from build123d import *

# Parameters (mm, degrees)
F1_DEPTH = 4.7625
F2_R     = 10


# Not quite as in the source:
# - a feature names something its author has since deleted; it is built from what else it names


with BuildPart() as f1:
    # F0 (on Top) → F1 (new body)
    with BuildSketch(Plane.XY):
        with BuildLine():
            ThreePointArc((-6.35, 0), (-4.4901280605, 4.4901280605), (0, 6.35))
            Line((0, 6.35), (-12.4931629071, 6.35))
            ThreePointArc((-12.4931629071, 6.35), (-13.6287381062, 3.2648303256), (-14.0143362106, 0))
            Line((-14.0143362106, 0), (-6.35, 0))
        make_face()
        with BuildLine():
            ThreePointArc((0, 6.35), (4.4901280605, 4.4901280605), (6.35, 0))
            Line((6.35, 0), (14.0143362106, 0))
            ThreePointArc((14.0143362106, 0), (13.6287381062, 3.2648303256), (12.4931629071, 6.35))
            Line((12.4931629071, 6.35), (0, 6.35))
        make_face()
        with BuildLine():
            Line((12.4931629071, -6.35), (0, -6.35))
            Line((0, -6.35), (0, -14.0143362106))
            ThreePointArc((0, -14.0143362106), (7.3283894713, -11.9455567966), (12.4931629071, -6.35))
        make_face()
        with BuildLine():
            Line((0, -14.0143362106), (0, -6.35))
            Line((0, -6.35), (-12.4931629071, -6.35))
            ThreePointArc((-12.4931629071, -6.35), (-7.3283894713, -11.9455567966), (0, -14.0143362106))
        make_face()
        with BuildLine():
            Line((-12.4931629071, -6.35), (0, -6.35))
            ThreePointArc((0, -6.35), (-4.4901280605, -4.4901280605), (-6.35, 0))
            Line((-6.35, 0), (-14.0143362106, 0))
            ThreePointArc((-14.0143362106, 0), (-13.6287381062, -3.2648303256), (-12.4931629071, -6.35))
        make_face()
        with BuildLine():
            Line((-27.86051193, -6.35), (-12.4931629071, -6.35))
            ThreePointArc((-12.4931629071, -6.35), (-13.6287381062, -3.2648303256), (-14.0143362106, 0))
            Line((-14.0143362106, 0), (-28.575, 0))
            ThreePointArc((-28.575, 0), (-28.395816183, -3.1950349451), (-27.86051193, -6.35))
        make_face()
        with BuildLine():
            ThreePointArc((12.4931629071, 6.35), (13.6287381062, 3.2648303256), (14.0143362106, 0))
            Line((14.0143362106, 0), (28.575, 0))
            ThreePointArc((28.575, 0), (28.395816183, 3.1950349451), (27.86051193, 6.35))
            Line((27.86051193, 6.35), (12.4931629071, 6.35))
        make_face()
        with BuildLine():
            Line((0, 14.0143362106), (0, 6.35))
            Line((0, 6.35), (12.4931629071, 6.35))
            ThreePointArc((12.4931629071, 6.35), (7.3283894713, 11.9455567966), (0, 14.0143362106))
        make_face()
        with BuildLine():
            Line((-12.4931629071, 6.35), (0, 6.35))
            Line((0, 6.35), (0, 14.0143362106))
            ThreePointArc((0, 14.0143362106), (-7.3283894713, 11.9455567966), (-12.4931629071, 6.35))
        make_face()
        with BuildLine():
            Line((-24.9023895556, -14.0143362106), (0, -14.0143362106))
            ThreePointArc((0, -14.0143362106), (-7.3283894713, -11.9455567966), (-12.4931629071, -6.35))
            Line((-12.4931629071, -6.35), (-27.86051193, -6.35))
            ThreePointArc((-27.86051193, -6.35), (-26.6583280736, -10.2890315054), (-24.9023895556, -14.0143362106))
        make_face()
        with BuildLine():
            Line((24.9023895556, 14.0143362106), (0, 14.0143362106))
            ThreePointArc((0, 14.0143362106), (7.3283894713, 11.9455567966), (12.4931629071, 6.35))
            Line((12.4931629071, 6.35), (27.86051193, 6.35))
            ThreePointArc((27.86051193, 6.35), (26.6583280736, 10.2890315054), (24.9023895556, 14.0143362106))
        make_face()
        with BuildLine():
            Line((14.0143362106, 0), (6.35, 0))
            ThreePointArc((6.35, 0), (4.4901280605, -4.4901280605), (0, -6.35))
            Line((0, -6.35), (12.4931629071, -6.35))
            ThreePointArc((12.4931629071, -6.35), (13.6287381062, -3.2648303256), (14.0143362106, 0))
        make_face()
        with BuildLine():
            ThreePointArc((-14.0143362106, 0), (-13.6287381062, 3.2648303256), (-12.4931629071, 6.35))
            Line((-12.4931629071, 6.35), (-27.86051193, 6.35))
            ThreePointArc((-27.86051193, 6.35), (-28.395816183, 3.1950349451), (-28.575, 0))
            Line((-28.575, 0), (-14.0143362106, 0))
        make_face()
        with BuildLine():
            ThreePointArc((-12.4931629071, 6.35), (-7.3283894713, 11.9455567966), (0, 14.0143362106))
            Line((0, 14.0143362106), (-24.9023895556, 14.0143362106))
            ThreePointArc((-24.9023895556, 14.0143362106), (-26.6583280736, 10.2890315054), (-27.86051193, 6.35))
            Line((-27.86051193, 6.35), (-12.4931629071, 6.35))
        make_face()
        with BuildLine():
            Line((28.575, 0), (14.0143362106, 0))
            ThreePointArc((14.0143362106, 0), (13.6287381062, -3.2648303256), (12.4931629071, -6.35))
            Line((12.4931629071, -6.35), (27.86051193, -6.35))
            ThreePointArc((27.86051193, -6.35), (28.395816183, -3.1950349451), (28.575, 0))
        make_face()
        with BuildLine():
            ThreePointArc((12.4931629071, -6.35), (7.3283894713, -11.9455567966), (0, -14.0143362106))
            Line((0, -14.0143362106), (24.9023895556, -14.0143362106))
            ThreePointArc((24.9023895556, -14.0143362106), (26.6583280736, -10.2890315054), (27.86051193, -6.35))
            Line((27.86051193, -6.35), (12.4931629071, -6.35))
        make_face()
    extrude(amount=F1_DEPTH)

    # F2
    f2_edges = [f1.edges().sort_by_distance(p)[0] for p in [
        (24.90239, 14.014336, 2.38125),
        (-24.90239, 14.014336, 2.38125),
        (24.90239, -14.014336, 2.38125),
        (-24.90239, -14.014336, 2.38125),
    ]]
    fillet(f2_edges, radius=F2_R)


solid = f1.part
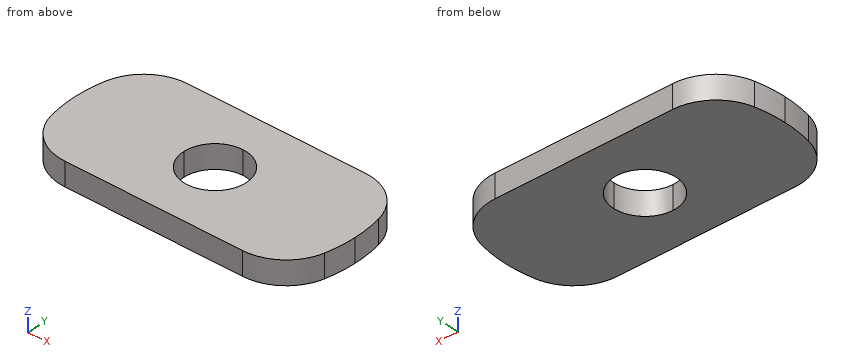
CAD build for the part. Positions are in the model's coordinates, mm. Coordinates: 2 decimals unless noted, no trailing zeros. Write each loop counter-clockwise with the first axis right and the second up, starting at its lowest first coordinate (ties: lowest second). Pieces come first, ordered by that corner, then holes. Notation, with made-up numbers: M 55.25,26 L 60.25,26 A26 ccw 60.25,65 Z; hole C 62.25,65.25 d5. An arc over 180 degrees is marked long. Return JSON: item names as keys, results as strings.
Item 1: Drop flat-ended pins along their axis: pin 1 Ø1 at (y, z) = (-11, 1.5) entering from +X; pin 2 Ø5 at (x, y) = (4.5, -1.5) entering from +Z; pin 3 Ø1.5 at (x, z) = (-21.5, 0.5) entering from -Y. Give the stop position or say it passes through.
Findings below:
{"pin 1": "stops at x = 25.75", "pin 2": "stops at z = 4.76", "pin 3": "stops at y = -13.67"}
Item 2: Slice it at B-B, the plane y = 1.75. Write the cut outline in (x, z), and give its area (3 significant figures).
Findings below:
{"outline": "M -28.52,0 L -6.1,0 L -6.1,4.76 L -28.52,4.76 Z; M 6.1,0 L 28.52,0 L 28.52,4.76 L 6.1,4.76 Z", "area": "214 mm2"}
Item 3: Slice it at A-A, the plane y = -1.25. Write the cut outline in (x, z), and give its area (3 significant figures).
Findings below:
{"outline": "M -28.55,0 L -6.23,0 L -6.23,4.76 L -28.55,4.76 Z; M 6.23,0 L 28.55,0 L 28.55,4.76 L 6.23,4.76 Z", "area": "213 mm2"}
Item 4: Probe line 1 (X direction, y = 3.75, z = 1.65); line 2 (X direction, y = -5.5, z = 0.85); line 3 (X direction, y = 11.75, z = 3.3). List the from-to ranges inside material, lowest first. Write a range as from..to.
Findings below:
{"line 1": "x = -28.33..-5.12, 5.12..28.33", "line 2": "x = -28.04..-3.17, 3.17..28.04", "line 3": "x = -24.47..24.47"}
